```python
from build123d import *

# Parameters (mm, degrees)
F2_R      = 6.35
F4_DEPTH  = 609.6
F3_R      = 6.35
F5_DEPTH  = 609.6
F1_R      = 6.35
F6_DEPTH  = 609.6
F7_W      = 155.56
F7_H      = 155.56
F8_DEPTH  = 25.4
F9_W      = 155.56
F9_H      = 155.56
F9_W_2    = 130.16
F9_H_2    = 130.16
F11_DEPTH = 38
F12_R     = 4.7625
F13_DEPTH = 1219.2


with BuildPart() as f4:
    # F2 (on Front) → F4 (new body, symmetric)
    with BuildSketch(Plane.XZ):
        Circle(F2_R)
    extrude(amount=F4_DEPTH, both=True)

    # F3 (on Right) → F5 (join, symmetric)
    with BuildSketch(Plane.YZ):
        Circle(F3_R)
    extrude(amount=F5_DEPTH, both=True)

    # F1 (on Top) → F6 (join, symmetric)
    with BuildSketch(Plane.XY):
        Circle(F1_R)
    extrude(amount=F6_DEPTH, both=True)

    # F7 (on face) → F8 (join)
    with BuildSketch(Plane.XZ.offset(609.6)):
        Rectangle(F7_W, F7_H)
    extrude(amount=-F8_DEPTH)

    # F9 (on face) → F11 (join)
    with BuildSketch(Plane.XZ.offset(609.6)):
        Rectangle(F9_W, F9_H)
        Rectangle(F9_W_2, F9_H_2, mode=Mode.SUBTRACT)
    extrude(amount=F11_DEPTH)

    # F12 (on face) → F13 (cut)
    with BuildSketch(Plane.XZ.offset(609.6)):
        Circle(F12_R)
    extrude(amount=-F13_DEPTH, mode=Mode.SUBTRACT)


solid = f4.part
```
Here's how the part is built. I have some questions about the finished solid (model axes, mm). A direction names the side the tool comes from. Give positions to 0.01 mm unless a question says otherwise; leave off trailing zeros. Write each loop counter-clockwise with the first axis right and the second up, starting at its lowest first coordinate (ties: lowest second). Pieces come first, ordered by that corner, then holes. Notation, with made-up numbers: M 87.25,87.5 L 101.25,87.5 A29 cw 101.25,113.5 Z; hole C -13.5,75.5 d5. An arc over 180 degrees is marked long. Put each result on its own line as item: value. Start each with the question number.
Item 1: If we section it at B-B, the plane x = 290.5: Write out the boundary of the cut face in (y, z), then the cut area to 3 significant figures.
Item 2: On a 3-axis mill with a long thin cutter (end or side, diameter ignored), from which of +Z, -Z, +X, -X, +Y, -Y can I reach the whole of each face in a straight line? I mean faces 1 (the flat face through (-70, -647.6, 1)), 2 (the flat face through (-1, -628, -65.08)). Say none if no direction works.
Item 3: I need wall thicknesses on L1, parallel to Z at x = 0, y = 16. Which ranges of the line are inside material? Lowest first, please. Write a range as from..to.
Item 4: Will this pin go through, and if not, where does the flat tip stop? pin 1 (5.5 mm diameter, centred on x = 0, z = 0, fed in from +Y) (1 decimal).
Item 5: Thinking about a two-plate mould opening in X: for faces 3 (the flat face through (-77.78, -615, -1)), 4 (the flat face through (-65.08, -628, -1)), 5 (the flat face through (-1, -615, -77.78)), which applies, +X half, -X half, draft (parallel to the pull), parting line (faces both ways), or undercut?
Values:
1. outline: C 0,0 d12.7
1. area: 127 mm²
2. face 1: +Z, -Z, +X, -X, -Y
2. face 2: -Y
3. L1: -6.35..-4.76, 4.76..6.35
4. pin 1: through
5. face 3: -X half
5. face 4: undercut
5. face 5: draft
